Geometry: final body of the model. Coordinates: model frame, mm. Give positions to 0.01 mm unless a question says otherwise; leave off trailing zeros. Loops run counter-clockwise (first coordinate to the right, second up) from the corner with the lowest first, then second, coordinate; pieces in that order, holes last.
1. Section B-B, the plane z = 1.25. Output: boundary loops of the cut face in (x, y).
2. Material intervals for line 1 along X through (y, z) = (0, 8.25); line 2 along Y through (x, z) = (1, 9); line 3 along Y through (x, z) = (0.7, 4.75), sorted ascending.
3. First-contact query: P1, Ø2, axis at x = -2, z = 1, coming from the -Y side; P2, Ø2, axis at x = 1.5, z = 5.5, coming from the +Y side. Flat tips, straight axial feed; report the tip coordinate or a pass-through.
4. Section A-A, the plane y = 0. Output: boundary loops of the cut face in (x, z), then the cut area to 3 significant figures.
5. Draft query along Y for faces 1 (the face through (0.769, 1.003, 4.93)), 2 (the face through (-0.03, -1.42, 0)), 3 (the face through (-1.394, -2.37, 4.938)). Return one class per face: +Y half, -Y half, draft (parallel to the pull), parting line (faces both ways), or undercut.
Autodesk Fusion 360 part; units mm, degrees
sketch "Skizze1" plane through (0, 0, 0) normal (0, 0, 1) x (1, 0, 0)
  line L0 (2.75, 1.5877) -> (0, 3.1754)
  line L1 (0, 3.1754) -> (-2.75, 1.5877)
  line L2 (-2.75, 1.5877) -> (-2.75, -1.5877)
  line L3 (-2.75, -1.5877) -> (0, -3.1754)
  line L4 (0, -3.1754) -> (2.75, -1.5877)
  line L5 (2.75, -1.5877) -> (2.75, 1.5877)
  dimension "d1" = 5.5
extrude "Extrusion1" add sketch "Skizze1" along normal blind 10
sketch "Skizze2" plane through (0, 0, 0) normal (1, 0, 0) x (0, 0, -1)
  line L0 (-10, 1.5877) -> (-10, 3.1754)
  line L1 (0, 1.5877) -> (0, 3.1754)
  line L2 (0, 3.1754) -> (-10, 3.1754)
  line L3 (2, 0.1754) -> (-1.5, 3.6754)
  line L4 (-1.5, 3.6754) -> (2, 3.6754)
  line L5 (2, 3.6754) -> (2, 0.1754)
  line L6 (-8.5, 3.6754) -> (-12, 3.6754)
  line L7 (-12, 3.6754) -> (-12, 0.1754)
  line L8 (-12, 0.1754) -> (-8.5, 3.6754)
  dimension "d4" = 45
  dimension "d5" = 45
  dimension "d6" = 2
  dimension "d7" = 2
  dimension "d8" = 3.5
  dimension "d9" = 0.5
revolve "Drehen1" cut sketch "Skizze2" angle 360 about axis through (0, 0, 1.75) along (0, 0, 1)
hole "Bohrung1" at (0, 0, 10) direction (0, 0, -1) diameter 2.529 end through all
Answers below:
1. outline: (-2.75, -1.59) - (0, -3.18) - (2.75, -1.59) - (2.75, 1.59) - (0, 3.18) - (-2.75, 1.59) - close; hole circle Ø2.53 at (0, 0)
2. line 1: x = -2.75 to -1.26, 1.26 to 2.75
2. line 2: y = -2.6 to -0.77, 0.77 to 2.6
2. line 3: y = -2.77 to -1.05, 1.05 to 2.77
3. P1: stops at y = -2.6
3. P2: stops at y = 2.89
4. outline: (-2.75, 0.57) - (-2.18, 0) - (-1.26, 0) - (-1.26, 10) - (-2.18, 10) - (-2.75, 9.43) - close; (1.26, 0) - (2.18, 0) - (2.75, 0.57) - (2.75, 9.43) - (2.18, 10) - (1.26, 10) - close
4. area: 29.0 mm2
5. face 1: undercut
5. face 2: draft
5. face 3: -Y half
